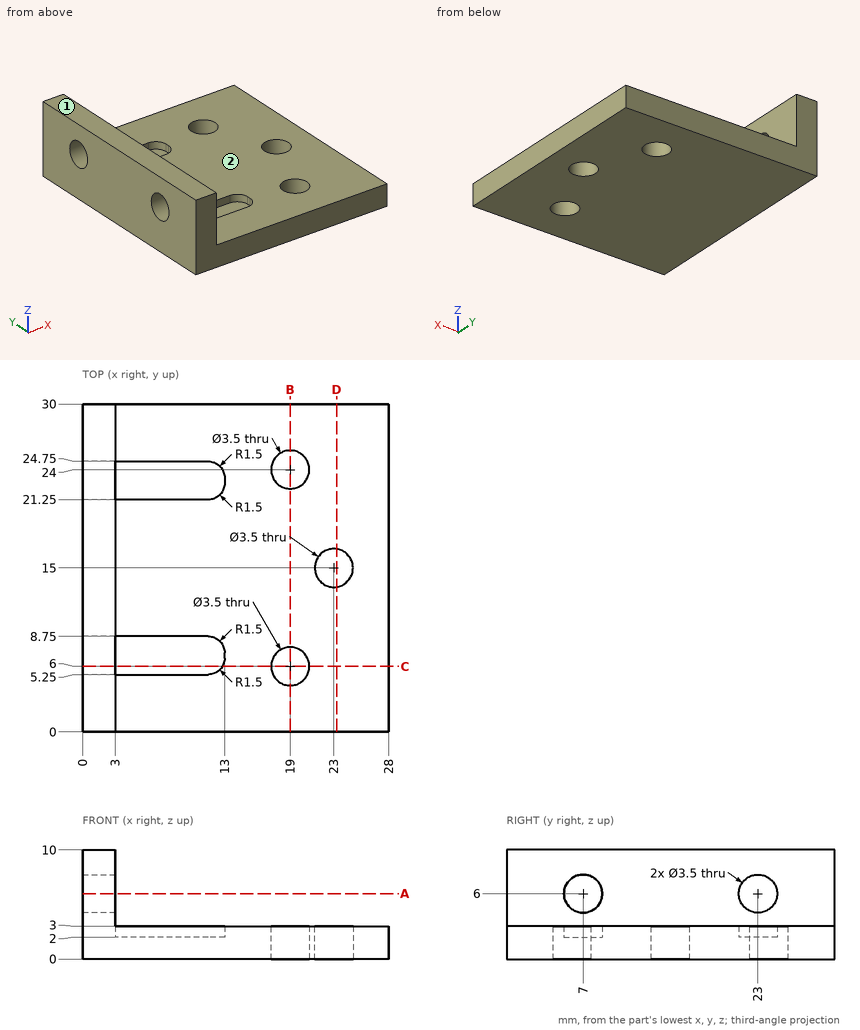
Job drawing, mm, ordinate dimensions from the low corner. One solid piece. A direction names the side the tool comes from. Coordinates: 2 decimals unless noted, no trailing zeros. Write each loop counter-clockwise with the first axis right and the second up, starting at its lowest first coordinate (ties: lowest second). Pieces come first, ordered by that corner, then holes. Notation, with made-up numbers: (80.25, 16.5) -> (95.25, 16.5) arc R11 ccw to (95.25, 24.5) -> close; hole circle Ø3 at (-9, -18). An arc over 180 degrees is marked (long way). Use CSV: the item, a comma, the result in double quotes. Start each with the question number.
Item 1: Wall check: probe 1 along Y at (x, z) = (19, 1.85); probe 2 along Y at (x, z) = (2.3, 6); probe 3 along X at (y, z) = (28.5, 8.5). Give the ranges that are in metal, low to high.
Item 2: Tool access for the marked faces 1 and 2: list every direction of +Z, -Z, +X, -X, +Y, -Y with a clear straight run to the whole face (end or side of a thin tool).
Item 3: Band-saw the part on A-A, the plane z = 6. Write the cut outline in (x, y), plus the area to 3 significant figures.
Item 4: Band-saw the part on D-D, the plane x = 23.25. Write the cut outline in (y, z).
Item 5: Band-saw the part on B-B, the plane x = 19. Write the cut outline in (y, z), plus the area to 3 significant figures.
Item 6: Drop flat-ended pins along their axis: P1, Ø5, axis at x = 25, y = 16.5, coming from the +Z side; P2, Ø1.8, axis at x = 6, y = 23, coming from the +Z side. Give the stop position or say it passes through.
Item 7: Band-saw the part on C-C, the plane y = 6. Write the cut outline in (x, z).
Response values:
1,probe 1,"y = 0 to 4.25, 7.75 to 22.25, 25.75 to 30"
1,probe 2,"y = 0 to 5.25, 8.75 to 21.25, 24.75 to 30"
1,probe 3,"x = 0 to 3"
2,face 1,"+Z, +X, -X, +Y, -Y"
2,face 2,"+Z, +X, +Y, -Y"
3,outline,"(0, 0) -> (3, 0) -> (3, 5.25) -> (0, 5.25) -> close; (0, 8.75) -> (3, 8.75) -> (3, 21.25) -> (0, 21.25) -> close; (0, 24.75) -> (3, 24.75) -> (3, 30) -> (0, 30) -> close"
3,area,"69.0 mm2"
4,outline,"(0, 0) -> (13.27, 0) -> (13.27, 3) -> (0, 3) -> close; (16.73, 0) -> (30, 0) -> (30, 3) -> (16.73, 3) -> close"
5,outline,"(0, 0) -> (4.25, 0) -> (4.25, 3) -> (0, 3) -> close; (7.75, 0) -> (22.25, 0) -> (22.25, 3) -> (7.75, 3) -> close; (25.75, 0) -> (30, 0) -> (30, 3) -> (25.75, 3) -> close"
5,area,"69.0 mm2"
6,P1,"stops at z = 3"
6,P2,"stops at z = 2"
7,outline,"(0, 0) -> (17.25, 0) -> (17.25, 3) -> (12.8, 3) -> (12.8, 2) -> (3, 2) -> (3, 4.56) -> (0, 4.56) -> close; (0, 7.44) -> (3, 7.44) -> (3, 10) -> (0, 10) -> close; (20.75, 0) -> (28, 0) -> (28, 3) -> (20.75, 3) -> close"
